Verification items for the finished model (mm, model axes). A direction names the side the tool comes from. Give positions to 0.01 mm unless a question says otherwise; leave off trailing zeros. Order: outer loops, then holes, each group sorted by start corner. A loop starts at its lowest first (then second) coordinate and runs counter-clockwise, first axis right, second up. Notation, with made-up numbers: (63, 36.5) - (118, 36.5) arc R8 ccw to (118, 47.5) - close; hole circle Ø10 at (29.25, 47.25). An arc over 180 degrees is marked (long way). Answer as a JSON object with one key per item and string values.
```python
from build123d import *

# Parameters (mm, degrees)
F0_W      = 2000
F0_H      = 1000
F1_DEPTH  = 25
F2_W      = 100
F2_H      = 100
F3_DEPTH  = 700
F4_R      = 25
F5_DEPTH  = 2819
F6_R      = 25
F7_DEPTH  = 2080
F8_R      = 25
F9_DEPTH  = 773
F10_R     = 25
F11_DEPTH = 1331
F12_R     = 25
F13_DEPTH = 1200
F14_R     = 25
F15_DEPTH = 1300
F16_DEPTH = 338
F17_R     = 25
F18_DEPTH = 1300
F19_R     = 10


with BuildPart() as f1:
    # F0 (on Front) → F1 (new body)
    with BuildSketch(Plane.XZ):
        with Locations((1000, 500)):
            Rectangle(F0_W, F0_H)
    extrude(amount=F1_DEPTH)

    # F2 (on face) → F3 (join)
    with BuildSketch(Plane(origin=(0, 0, 0), x_dir=(-1, 0, 0), z_dir=(0, 1, 0))):
        with Locations((-1900, 100)):
            Rectangle(F2_W, F2_H)
        with Locations((-100, 100)):
            Rectangle(F2_W, F2_H)
        with Locations((-1900, 900)):
            Rectangle(F2_W, F2_H)
        with Locations((-100, 900)):
            Rectangle(F2_W, F2_H)
    extrude(amount=F3_DEPTH)

    # F4 (on face) → F5 (cut)
    with BuildSketch(Plane(origin=(0, 0, 50), x_dir=(1, 0, 0), z_dir=(0, 0, -1))):
        with Locations((1900, -500)):
            Circle(F4_R)
    extrude(amount=-F5_DEPTH, mode=Mode.SUBTRACT)

    # F6 (on face) → F7 (cut)
    with BuildSketch(Plane.XY.offset(150)):
        with Locations((1900, 300)):
            Circle(F6_R)
    extrude(amount=F7_DEPTH, mode=Mode.SUBTRACT)

    # F8 (on face) → F9 (cut)
    with BuildSketch(Plane.XY.offset(150)):
        with Locations((1900, 100)):
            Circle(F8_R)
    extrude(amount=F9_DEPTH, mode=Mode.SUBTRACT)

    # F10 (on face) → F11 (cut)
    with BuildSketch(Plane.XY.offset(950)):
        with Locations((100, 475)):
            Circle(F10_R)
    extrude(amount=-F11_DEPTH, mode=Mode.SUBTRACT)

    # F12 (on face) → F13 (cut)
    with BuildSketch(Plane.XY.offset(950)):
        with Locations((100, 275)):
            Circle(F12_R)
    extrude(amount=-F13_DEPTH, mode=Mode.SUBTRACT)

    # F14 (on face) → F15 (cut)
    with BuildSketch(Plane.XY.offset(950)):
        with Locations((100, 75)):
            Circle(F14_R)
    extrude(amount=-F15_DEPTH, mode=Mode.SUBTRACT)

    # F6 (on face) → F16 (cut)
    with BuildSketch(Plane.XY.offset(150)):
        with Locations((1900, 300)):
            Circle(F6_R)
    extrude(amount=-F16_DEPTH, mode=Mode.SUBTRACT)

    # F17 (on face) → F18 (cut)
    with BuildSketch(Plane.XY.offset(950)):
        with Locations((1900, 100)):
            Circle(F17_R)
    extrude(amount=-F18_DEPTH, mode=Mode.SUBTRACT)

    # F19
    f19_edges = [f1.edges().sort_by_distance(p)[0] for p in [
        (1000, -25, 0),
        (0, -25, 500),
        (1000, -25, 1000),
        (2000, -25, 500),
    ]]
    fillet(f19_edges, radius=F19_R)


solid = f1.part
```
(1) Section check C-C (x = 100). Count the separate pieces of the cut face and the enclosed holes in it, then the cut area to 3 significant figures.
Computed values:
{"separate pieces": "7", "enclosed holes": "0", "area": "135,000 mm²"}
(2) Section check A-A (y = 655.5). Record the cut outline in (x, z).
Computed values:
{"outline": "(50, 50) - (150, 50) - (150, 150) - (50, 150) - close; (50, 850) - (150, 850) - (150, 950) - (50, 950) - close; (1850, 50) - (1950, 50) - (1950, 150) - (1850, 150) - close; (1850, 850) - (1950, 850) - (1950, 950) - (1850, 950) - close"}
(3) Material ranges on line 1 along Y through (x, z) = (100, 114); line 2 along Y through (x, z) = (1900, 903); line 3 along X through (y, z) = (146, 94.5), recorded low to high. Write a range as [from, to].
Computed values:
{"line 1": "y = [-25, 50], [100, 250], [300, 450], [500, 700]", "line 2": "y = [-25, 75], [125, 275], [325, 475], [525, 700]", "line 3": "x = [50, 150], [1850, 1950]"}
(4) Section check D-D (x = 669.5). Record the cut outline in (y, z).
Computed values:
{"outline": "(-25, 10) arc R10 ccw to (-15, 0) - (0, 0) - (0, 1000) - (-15, 1000) arc R10 ccw to (-25, 990) - close"}
(5) Gauge pin test, flat end, axial feed: pin 1 Ø4 at (x, z) = (1402.5, 489) entering from +Y. Record the tip position at first contact, or that the pin passes through.
Computed values:
{"pin 1": "stops at y = 0"}
(6) Release check for a two-part mould opening along X. For faces 4 (the cylindrical face through (80, 60, 101)), 5 (the flat face through (101, 345, 150)), 6 (the flat face through (1950, 345, 899)) record: pulls with the +X half, pulls with the -X half, needs draft (parallel to the pull), parting line crosses it, or undercut.
Computed values:
{"face 4": "undercut", "face 5": "needs draft", "face 6": "pulls with the +X half"}
(7) Section check B-B (z = 120). Record the cut outline in (x, y), then the cut area to 3 significant figures.
Computed values:
{"outline": "(0, -15) arc R10 ccw to (10, -25) - (1990, -25) arc R10 ccw to (2000, -15) - (2000, 0) - (1950, 0) - (1950, 700) - (1850, 700) - (1850, 0) - (150, 0) - (150, 700) - (50, 700) - (50, 0) - (0, 0) - close; hole circle Ø50 at (100, 75); hole circle Ø50 at (100, 275); hole circle Ø50 at (100, 475); hole circle Ø50 at (1900, 100); hole circle Ø50 at (1900, 300); hole circle Ø50 at (1900, 500)", "area": "178,000 mm²"}
(8) Access from +Z, -Z, +X, -X, +Y, -Y to the whole of each face (thin tool, end or side, straight path). Record for faces 1 (the flat face through (1850, 345, 899)), 2 (the flat face through (101, 345, 950)), 3 (the flat face through (1901, 345, 850)).
Computed values:
{"face 1": "+Z, -Z, +Y", "face 2": "+Z, +X, -X, +Y", "face 3": "+X, -X, +Y"}
